Design review of the part built by this model. Coordinates are the model's own, in mm. A direction names the side the tool comes from. Round coordinates to 2 decimals unless told otherwise and drop trailing zeros. Order: outer loops, then holes, each group sorted by start corner. A loop starts at its lowest first (then second) coordinate and runs counter-clockwise, first axis right, second up.
from build123d import *

# Parameters (mm, degrees)
SKETCH_1_W                       = 230
SKETCH_1_H                       = 150
EXTRUDE_1_DEPTH                  = 18
CUT_EXTRUDE_2_DEPTH              = 16
FILLET_1_R                       = 5
SKETCH_3_R                       = 2.5
CUT_EXTRUDE_4_DEPTH              = 19
SKETCH_5_W                       = 165
SKETCH_5_H                       = 100
CUT_EXTRUDE_5_DEPTH              = 19
CUT_EXTRUDE_8_REACH              = 20
SKETCH_7_R                       = 1.5
CUT_EXTRUDE_9_REACH              = 20
SKETCH_8_R                       = 5
CUT_EXTRUDE_10_REACH             = 20
SKETCH_6_W                       = 29
SKETCH_6_H                       = 4
CUT_EXTRUDE_11_REACH             = 20
SKETCH_6_3_W                     = 32
SKETCH_6_3_H                     = 4
CUT_EXTRUDE_11_DIRECTION_2_DEPTH = 1


with BuildPart() as part:
    # 草图1 → 凸台-拉伸1 (new body)
    with BuildSketch(Plane(origin=(0, 0, 0), x_dir=(1, 0, 0), z_dir=(0, 1, 0))):
        with Locations((115, 75)):
            Rectangle(SKETCH_1_W, SKETCH_1_H)
    extrude(amount=EXTRUDE_1_DEPTH)

    # 草图2 → 切除-拉伸2 (cut)
    with BuildSketch(Plane(origin=(0, 18, 0), x_dir=(1, 0, 0), z_dir=(0, 1, 0))):
        Polygon((2, 125.5), (2, 24.5), (15.5, 24.5), (15.5, 2), (214.5, 2), (214.5, 24.5), (228, 24.5), (228, 125.5), (214.5, 125.5), (214.5, 148), (15.5, 148), (15.5, 125.5), align=None)
    extrude(amount=-CUT_EXTRUDE_2_DEPTH, mode=Mode.SUBTRACT)

    # 圆角1
    fillet_1_edges = [part.edges().sort_by_distance(p)[0] for p in [
        (2, 10, -125.5),
        (15.5, 10, -125.5),
        (15.5, 10, -148),
        (214.5, 10, -148),
        (214.5, 10, -125.5),
        (228, 10, -125.5),
        (228, 10, -24.5),
        (214.5, 10, -24.5),
        (214.5, 10, -2),
        (15.5, 10, -2),
        (15.5, 10, -24.5),
        (2, 10, -24.5),
        (0, 9, -150),
        (230, 9, -150),
        (230, 9, 0),
        (0, 9, 0),
    ]]
    fillet(fillet_1_edges, radius=FILLET_1_R)

    # 草图3 → 切除-拉伸4 (cut, through all)
    with BuildSketch(Plane(origin=(0, 18, 0), x_dir=(1, 0, 0), z_dir=(0, 1, 0))):
        with Locations((8, 142)):
            Circle(SKETCH_3_R)
        with Locations((222.21463853, 142)):
            Circle(SKETCH_3_R)
        with Locations((8, 8.013915663)):
            Circle(SKETCH_3_R)
        with Locations((222, 8)):
            Circle(SKETCH_3_R)
    extrude(amount=-CUT_EXTRUDE_4_DEPTH, mode=Mode.SUBTRACT)

    # 草图5 → 切除-拉伸5 (cut, through all)
    with BuildSketch(Plane.XZ):
        with Locations((115, -75)):
            Rectangle(SKETCH_5_W, SKETCH_5_H)
    extrude(amount=-CUT_EXTRUDE_5_DEPTH, mode=Mode.SUBTRACT)

    # 草图7 → 切除-拉伸8 (cut, up to next)
    with BuildSketch(Plane.XZ, mode=Mode.PRIVATE) as cut_extrude_8_sk1:
        with Locations((27.5, -24)):
            Circle(SKETCH_7_R)
    cut_extrude_8_tool1 = extrude(cut_extrude_8_sk1.sketch, amount=-CUT_EXTRUDE_8_REACH, mode=Mode.PRIVATE) & part.part
    add(cut_extrude_8_tool1.solids().sort_by_distance((27.5, 0, -24))[0], mode=Mode.SUBTRACT)
    # 草图7 → 切除-拉伸8 (cut, up to next)
    with BuildSketch(Plane.XZ, mode=Mode.PRIVATE) as cut_extrude_8_sk2:
        with Locations((202.5, -126)):
            Circle(SKETCH_7_R)
    cut_extrude_8_tool2 = extrude(cut_extrude_8_sk2.sketch, amount=-CUT_EXTRUDE_8_REACH, mode=Mode.PRIVATE) & part.part
    add(cut_extrude_8_tool2.solids().sort_by_distance((202.5, 0, -126))[0], mode=Mode.SUBTRACT)
    # 草图7 → 切除-拉伸8 (cut, up to next)
    with BuildSketch(Plane.XZ, mode=Mode.PRIVATE) as cut_extrude_8_sk3:
        with Locations((27.5, -126)):
            Circle(SKETCH_7_R)
    cut_extrude_8_tool3 = extrude(cut_extrude_8_sk3.sketch, amount=-CUT_EXTRUDE_8_REACH, mode=Mode.PRIVATE) & part.part
    add(cut_extrude_8_tool3.solids().sort_by_distance((27.5, 0, -126))[0], mode=Mode.SUBTRACT)
    # 草图7 → 切除-拉伸8 (cut, up to next)
    with BuildSketch(Plane.XZ, mode=Mode.PRIVATE) as cut_extrude_8_sk4:
        with Locations((202.5, -24)):
            Circle(SKETCH_7_R)
    cut_extrude_8_tool4 = extrude(cut_extrude_8_sk4.sketch, amount=-CUT_EXTRUDE_8_REACH, mode=Mode.PRIVATE) & part.part
    add(cut_extrude_8_tool4.solids().sort_by_distance((202.5, 0, -24))[0], mode=Mode.SUBTRACT)

    # 草图8 → 切除-拉伸9 (cut, up to next)
    with BuildSketch(Plane.XZ, mode=Mode.PRIVATE) as cut_extrude_9_sk1:
        with Locations((14.5, -75)):
            Circle(SKETCH_8_R)
    cut_extrude_9_tool1 = extrude(cut_extrude_9_sk1.sketch, amount=-CUT_EXTRUDE_9_REACH, mode=Mode.PRIVATE) & part.part
    add(cut_extrude_9_tool1.solids().sort_by_distance((14.5, 0, -75))[0], mode=Mode.SUBTRACT)
    # 草图8 → 切除-拉伸9 (cut, up to next)
    with BuildSketch(Plane.XZ, mode=Mode.PRIVATE) as cut_extrude_9_sk2:
        with Locations((115, -11)):
            Circle(SKETCH_8_R)
    cut_extrude_9_tool2 = extrude(cut_extrude_9_sk2.sketch, amount=-CUT_EXTRUDE_9_REACH, mode=Mode.PRIVATE) & part.part
    add(cut_extrude_9_tool2.solids().sort_by_distance((115, 0, -11))[0], mode=Mode.SUBTRACT)
    # 草图8 → 切除-拉伸9 (cut, up to next)
    with BuildSketch(Plane.XZ, mode=Mode.PRIVATE) as cut_extrude_9_sk3:
        with Locations((215.5, -75)):
            Circle(SKETCH_8_R)
    cut_extrude_9_tool3 = extrude(cut_extrude_9_sk3.sketch, amount=-CUT_EXTRUDE_9_REACH, mode=Mode.PRIVATE) & part.part
    add(cut_extrude_9_tool3.solids().sort_by_distance((215.5, 0, -75))[0], mode=Mode.SUBTRACT)
    # 草图8 → 切除-拉伸9 (cut, up to next)
    with BuildSketch(Plane.XZ, mode=Mode.PRIVATE) as cut_extrude_9_sk4:
        with Locations((115, -139)):
            Circle(SKETCH_8_R)
    cut_extrude_9_tool4 = extrude(cut_extrude_9_sk4.sketch, amount=-CUT_EXTRUDE_9_REACH, mode=Mode.PRIVATE) & part.part
    add(cut_extrude_9_tool4.solids().sort_by_distance((115, 0, -139))[0], mode=Mode.SUBTRACT)

    # 草图6 → 切除-拉伸10 (cut, up to next)
    with BuildSketch(Plane.XZ, mode=Mode.PRIVATE) as cut_extrude_10_sk1:
        with Locations((52, -23)):
            Rectangle(SKETCH_6_W, SKETCH_6_H)
    cut_extrude_10_tool1 = extrude(cut_extrude_10_sk1.sketch, amount=-CUT_EXTRUDE_10_REACH, mode=Mode.PRIVATE) & part.part
    add(cut_extrude_10_tool1.solids().sort_by_distance((52, 0, -23))[0], mode=Mode.SUBTRACT)

    # 草图6<3> → 切除-拉伸11 (cut, up to next)
    with BuildSketch(Plane.XZ, mode=Mode.PRIVATE) as cut_extrude_11_sk1:
        with Locations((115.5, -23)):
            Rectangle(SKETCH_6_3_W, SKETCH_6_3_H)
    cut_extrude_11_tool1 = extrude(cut_extrude_11_sk1.sketch, amount=-CUT_EXTRUDE_11_REACH, mode=Mode.PRIVATE) & part.part
    add(cut_extrude_11_tool1.solids().sort_by_distance((115.5, 0, -23))[0], mode=Mode.SUBTRACT)

    # 草图6<3> → 切除-拉伸11 direction 2 (cut)
    with BuildSketch(Plane.XZ):
        with Locations((115.5, -23)):
            Rectangle(SKETCH_6_3_W, SKETCH_6_3_H)
    extrude(amount=CUT_EXTRUDE_11_DIRECTION_2_DEPTH, mode=Mode.SUBTRACT)


solid = part.part
1) To check wall thickness, follow line 1 along X through (y, z) = (12.75, -142); line 2 along Z through (x, y) = (27.5, 1.2); line 3 along X through (y, z) = (0.9, -126). State the ranges of each line that lie inside material, in increasing order.
Results:
line 1: x = 0 to 5.5, 10.5 to 15.5, 214.5 to 219.71, 224.71 to 230
line 2: z = -150 to -127.5, -124.5 to -25.5, -22.5 to 0
line 3: x = 0 to 26, 29 to 201, 204 to 230
2) The part is to be moulded in two halves that separate along X. For faces 1 (the face through (226.5, 9.89, -25.93)), 2 (the face through (1, 9, -2)), 3 (the face through (15.5, 10, -13)), 4 (the face through (228, 9, -1)), say which applies: released by +X, released by -X, zero draft, split by the parting line, or undercut.
Results:
face 1: undercut
face 2: released by -X
face 3: undercut
face 4: released by +X
3) Take a section at D-D on y = 12.75. State how many separate pieces and enclosed holes the cut face has, plus the area to 3 significant figures.
Results:
separate pieces: 1
enclosed holes: 5
area: 2,640 mm2
4) Take a section at C-C on z = -103. Give the boundary of the cut face in (x, y), plus the area to 3 significant figures.
Results:
outline: (0, 0) - (32.5, 0) - (32.5, 2) - (2, 2) - (2, 18) - (0, 18) - close; (197.5, 0) - (230, 0) - (230, 18) - (228, 18) - (228, 2) - (197.5, 2) - close
area: 194 mm2
5) Take a section at A-A on z = -75. Give the boundary of the cut face in (x, y).
Results:
outline: (0, 0) - (9.5, 0) - (9.5, 2) - (2, 2) - (2, 18) - (0, 18) - close; (19.5, 0) - (32.5, 0) - (32.5, 2) - (19.5, 2) - close; (197.5, 0) - (210.5, 0) - (210.5, 2) - (197.5, 2) - close; (220.5, 0) - (230, 0) - (230, 18) - (228, 18) - (228, 2) - (220.5, 2) - close
6) For faces 5 (the face through (214.5, 10, -137)), 6 (the face through (113, 9, -150)), list the 3-axis set-ups (+Z, -Z, +X, -X, +Y, -Y) from which the entire face can be reached by the end or side of a thin tool; tool diameter is ignored.
Results:
face 5: +Y
face 6: -Z, +X, -X, +Y, -Y
7) Take a section at B-B on x = 56.5. Give the boundary of the cut face in (y, z), plus the area to 3 significant figures.
Results:
outline: (0, -150) - (18, -150) - (18, -148) - (2, -148) - (2, -125) - (0, -125) - close; (0, -21) - (2, -21) - (2, -2) - (18, -2) - (18, 0) - (0, 0) - close
area: 156 mm2
8) Clearance check with a flat-ended pin moving along its axis: P1, Ø12, axis at x = 115.5, z = -16, coming from the +Y side. State where the tip first meets the part, or that it passes through.
Results:
P1: stops at y = 2
